```python
from build123d import *

# Parameters (mm, degrees)
SKETCH1_R           = 40
SKETCH1_R_2         = 30
BOSS_EXTRUDE2_DEPTH = 20
SKETCH2_W           = 120
SKETCH2_H           = 80
BOSS_EXTRUDE3_DEPTH = 15
SKETCH3_R           = 15
CUT_EXTRUDE1_DEPTH  = 37
SKETCH7_W           = 20
SKETCH7_H           = 35
BOSS_EXTRUDE5_DEPTH = 80
BOSS_EXTRUDE6_DEPTH = 20
SKETCH9_R           = 16
CUT_EXTRUDE2_DEPTH  = 20


with BuildPart() as part:
    # Sketch1 → Boss-Extrude2 (new body)
    with BuildSketch(Plane(origin=(0, 0, 0), x_dir=(1, 0, 0), z_dir=(0, 1, 0))):
        with Locations(Location((0, 0, 0), (0, 0, 270))):
            Circle(SKETCH1_R)
        with Locations(Location((0, 0, 0), (0, 0, 270))):
            Circle(SKETCH1_R_2, mode=Mode.SUBTRACT)
    extrude(amount=BOSS_EXTRUDE2_DEPTH)

    # Sketch2 → Boss-Extrude3 (add)
    with BuildSketch(Plane(origin=(0, 20, 0), x_dir=(1, 0, 0), z_dir=(0, 1, 0))):
        Rectangle(SKETCH2_W, SKETCH2_H)
    extrude(amount=BOSS_EXTRUDE3_DEPTH)

    # Sketch3 → Cut-Extrude1 (cut)
    with BuildSketch(Plane.XZ.offset(-20)):
        with Locations(Location((0, 0, 0), (0, 0, 270))):
            Circle(SKETCH3_R)
    extrude(amount=-CUT_EXTRUDE1_DEPTH, mode=Mode.SUBTRACT)

    # Sketch7 → Boss-Extrude5 (add)
    with BuildSketch(Plane.XY.offset(40)):
        with Locations((50, 52.5)):
            Rectangle(SKETCH7_W, SKETCH7_H)
    boss_extrude5 = extrude(amount=-BOSS_EXTRUDE5_DEPTH)

    # Sketch8 → Boss-Extrude6 (add)
    with BuildSketch(Plane.ZY.offset(-40)):
        with BuildLine():
            Line((40, 70), (-40, 70))
            ThreePointArc((-40, 70), (0, 110), (40, 70))
        make_face()
    boss_extrude6 = extrude(amount=-BOSS_EXTRUDE6_DEPTH)

    # Sketch9 → Cut-Extrude2 (cut)
    with BuildSketch(Plane(origin=(60, 0, 0), x_dir=(0, 0, -1), z_dir=(1, 0, 0))):
        with Locations((0, 70)):
            Circle(SKETCH9_R)
    cut_extrude2 = extrude(amount=-CUT_EXTRUDE2_DEPTH, mode=Mode.SUBTRACT)

    # Mirror1: Boss-Extrude5, Boss-Extrude6, Cut-Extrude2 across plane
    add(boss_extrude5.mirror(Plane(origin=(0, 0, 0), x_dir=(0, 0, 1), z_dir=(1, 0, 0))))
    add(boss_extrude6.mirror(Plane(origin=(0, 0, 0), x_dir=(0, 0, 1), z_dir=(1, 0, 0))))
    add(cut_extrude2.mirror(Plane(origin=(0, 0, 0), x_dir=(0, 0, 1), z_dir=(1, 0, 0))), mode=Mode.SUBTRACT)


solid = part.part
```
The model under review builds one solid part; all positions refer to its coordinate system, in mm. A direction names the side the tool comes from. Give positions to 0.01 mm unless a question says otherwise; leave off trailing zeros. Loops run counter-clockwise (first coordinate to the right, second up) from the corner with the lowest first, then second, coordinate; pieces in that order, holes last. Notation, with made-up numbers: (45.25, 45.25) -> (95.25, 45.25) arc R8 ccw to (95.25, 60.25) -> close; hole circle Ø6 at (63, -5). An arc over 180 degrees is marked (long way). Use CSV: the item, a comma, the result in double quotes.
1. Consider section D-D, the plane x = 48.5. Write out the cut boundary in (y, z).
Result:
outline,"(20, -40) -> (70, -40) arc R40 ccw to (70, 40) -> (20, 40) -> close; hole circle Ø32 at (70, 0)"
2. For P1, Ø12, axis at y = 12.5, z = 1, coming from the +X side; P2, Ø18, axis at x = 4, z = 1, coming from the -Y side; P3, Ø2, axis at x = 5.5, z = 26.5, coming from the -Y side, all flat-tipped, find the tip position at first contact; note any pin that passes through.
Result:
P1,"stops at x = 40"
P2,"passes through"
P3,"stops at y = 20"
3. Consider section A-A, the plane z = 0. Write out the cut boundary in (x, y), then the cut area to 3 significant figures.
Result:
outline,"(-60, 20) -> (-40, 20) -> (-40, 0) -> (-30, 0) -> (-30, 20) -> (-15, 20) -> (-15, 35) -> (-40, 35) -> (-40, 54) -> (-60, 54) -> close; (-60, 86) -> (-40, 86) -> (-40, 110) -> (-60, 110) -> close; (15, 20) -> (30, 20) -> (30, 0) -> (40, 0) -> (40, 20) -> (60, 20) -> (60, 54) -> (40, 54) -> (40, 35) -> (15, 35) -> close; (40, 86) -> (60, 86) -> (60, 110) -> (40, 110) -> close"
area,"3,470 mm²"
4. To check wall thickness, follow probe 1 along X at (y, z) = (52, -27); probe 2 along X at (y, z) = (7.5, 0); probe 3 along Y at (x, z) = (51.5, 0). State the ranges of each line that lie inside material, in increasing order. Write a range as from..to.
Result:
probe 1,"x = -60..-40, 40..60"
probe 2,"x = -40..-30, 30..40"
probe 3,"y = 20..54, 86..110"
5. Consider section B-B, the plane y = 51. Write out the cut boundary in (x, z).
Result:
outline,"(-60, -40) -> (-40, -40) -> (-40, 40) -> (-60, 40) -> close; (40, -40) -> (60, -40) -> (60, 40) -> (40, 40) -> close"
6. Machinability: for faces 1 (the face through (-44, 20, -1)), 2 (the face through (1.32, 9.86, -29.97)), 3 (the face through (43, 20, -1)), which of the approach directions +Z, -Z, +X, -X, +Y, -Y give a long, thin tool a straight path to every point of the face, cutting with its end or side? Answer none if there is none.
Result:
face 1,"-X, -Y"
face 2,"-Y"
face 3,"+X, -Y"
7. Consider section C-C, the plane x = 32. Write out the cut boundary in (y, z).
Result:
outline,"(0, -24) -> (20, -24) -> (20, -40) -> (35, -40) -> (35, 40) -> (20, 40) -> (20, 24) -> (0, 24) -> close"
8. The part is to be moulded in two halves that separate along Z. For faces 4 (the face through (50.14, 85.864, 2.083)), 5 (the face through (60, 55.6, -8.3)), 6 (the face through (1, 34, -40)), 7 (the face through (1, 34, 40)), say which applies: +Z half, -Z half, draft (parallel to the pull), parting line (faces both ways), or undercut.
Result:
face 4,"undercut"
face 5,"draft"
face 6,"-Z half"
face 7,"+Z half"
